Autodesk Inventor part; units mm, degrees
ref_plane "YZ Plane" through (0, 0, 0) normal (1, 0, 0) x (0, 1, 0)
ref_plane "XZ Plane" through (0, 0, 0) normal (0, 1, 0) x (-1, 0, 0)
ref_plane "XY Plane" through (0, 0, 0) normal (0, 0, 1) x (1, 0, 0)
sketch "Skizze1" plane through (0, 0, 0) normal (0, 0, 1) x (1, 0, 0)
  line L0 (-15.4, 0) -> (15.4, 0)
  line L1 (0, -42) -> (0, 42)
  line L2 (11, -30) -> (-11, -30)
  line L3 (-11, -30) -> (-11, 30)
  line L4 (-11, 30) -> (11, 30)
  line L5 (11, 30) -> (11, -30)
  line L6 (11, -30) -> (-11, 30) construction
  line L7 (-11, -30) -> (11, 30) construction
  point P0 (0, 0)
  dimension "d0" = 60
  dimension "d1" = 22
extrude "Extrusion1" add sketch "Skizze1" along normal blind 3
sketch "Skizze2" plane through (0, 0, 3) normal (0, 0, 1) x (1, 0, 0)
  line L0 (11, 30) -> (-11, 30)
  line L1 (-11, 30) -> (-11, -30)
  line L2 (-11, -30) -> (11, -30)
  line L3 (11, -30) -> (11, 30)
  line L4 (-17.5, 0) -> (17.5, 0)
  line L5 (0, -42) -> (0, 42)
  line L6 (3.1579, -20) -> (-3.1579, -20)
  line L7 (-3.1579, -20) -> (-3.1579, 20)
  line L8 (-3.1579, 20) -> (3.1579, 20)
  line L9 (3.1579, 20) -> (3.1579, -20)
  line L10 (3.1579, -20) -> (-3.1579, 20) construction
  line L11 (-3.1579, -20) -> (3.1579, 20) construction
  point P0 (0, 0)
  point P1 (0, 20)
  point P2 (0, -20)
  dimension "d4" = 40
hole "Bohrung1" at (0, 20, 3) at (0, -20, 3) direction (0, 0, -1) diameter 5.2 end through all
fillet "Rundung1" radius 10 4 edges at (-11, 30, 1.5) (11, 30, 1.5) (11, -30, 1.5) (-11, -30, 1.5)
sketch "Skizze3" plane through (0, 0, 3) normal (0, 0, 1) x (1, 0, 0)
  point P0 (0, 0)
properties part number "24_0497_005"
Design review of the part built by this model. Coordinates are the model's own, in mm. Round coordinates to 2 decimals unless told otherwise and drop trailing zeros. Write each loop counter-clockwise with the first axis right and the second up, starting at its lowest first coordinate (ties: lowest second). Pieces come first, ordered by that corner, then holes. Notation, with made-up numbers: (-31, 65.5) - (-3, 65.5) arc R6 cw to (-3, 74.5) - close; hole circle Ø5 at (36, 13.5). An arc over 180 degrees is marked (long way). Use a Markdown table: item, result. Add a question column.
1. We need section B-B (z = 0.65). State the section outline as (x, y) points.
2. Mouldability with a two-part tool opening along X and no side actions: class faces 1 (the face through (-7.99, 27.15, 1.52)), 2 (the face through (-0.78, 17.52, 1.48)), 3 (the face through (0, 0, 3)) as +X half, -X half, draft (parallel to the pull), parting line (faces both ways), or undercut.
3. We need section D-D (y = 26). State the section outline as (x, z) points.
4. Wall thickness on probe 1 along Y at (x, z) = (0, 1); probe 2 along X at (y, z) = (-20, 0.7); probe 3 along Y at (x, z) = (-4.25, 2.9): over which ranges is each line inside the solid? List them lowest first.
5. We need section C-C (y = -21). State the section outline as (x, z) points.
6. We need section A-A (x = 0). State the section outline as (y, z) points, then the cut area to 3 significant figures.
Output:
| question | item | result |
|---|---|---|
| 1 | outline | (-11, -20) arc R10 ccw to (-1, -30) - (1, -30) arc R10 ccw to (11, -20) - (11, 20) arc R10 ccw to (1, 30) - (-1, 30) arc R10 ccw to (-11, 20) - close; hole circle Ø5.2 at (0, -20); hole circle Ø5.2 at (0, 20) |
| 2 | face 1 | -X half |
| 2 | face 2 | undercut |
| 2 | face 3 | draft |
| 3 | outline | (-9, 0) - (9, 0) - (9, 3) - (-9, 3) - close |
| 4 | probe 1 | y = -30 to -22.6, -17.4 to 17.4, 22.6 to 30 |
| 4 | probe 2 | x = -11 to -2.6, 2.6 to 11 |
| 4 | probe 3 | y = -29.46 to 29.46 |
| 5 | outline | (-10.95, 0) - (-2.4, 0) - (-2.4, 3) - (-10.95, 3) - close; (2.4, 0) - (10.95, 0) - (10.95, 3) - (2.4, 3) - close |
| 6 | outline | (-30, 0) - (-22.6, 0) - (-22.6, 3) - (-30, 3) - close; (-17.4, 0) - (17.4, 0) - (17.4, 3) - (-17.4, 3) - close; (22.6, 0) - (30, 0) - (30, 3) - (22.6, 3) - close |
| 6 | area | 149 mm2 |
